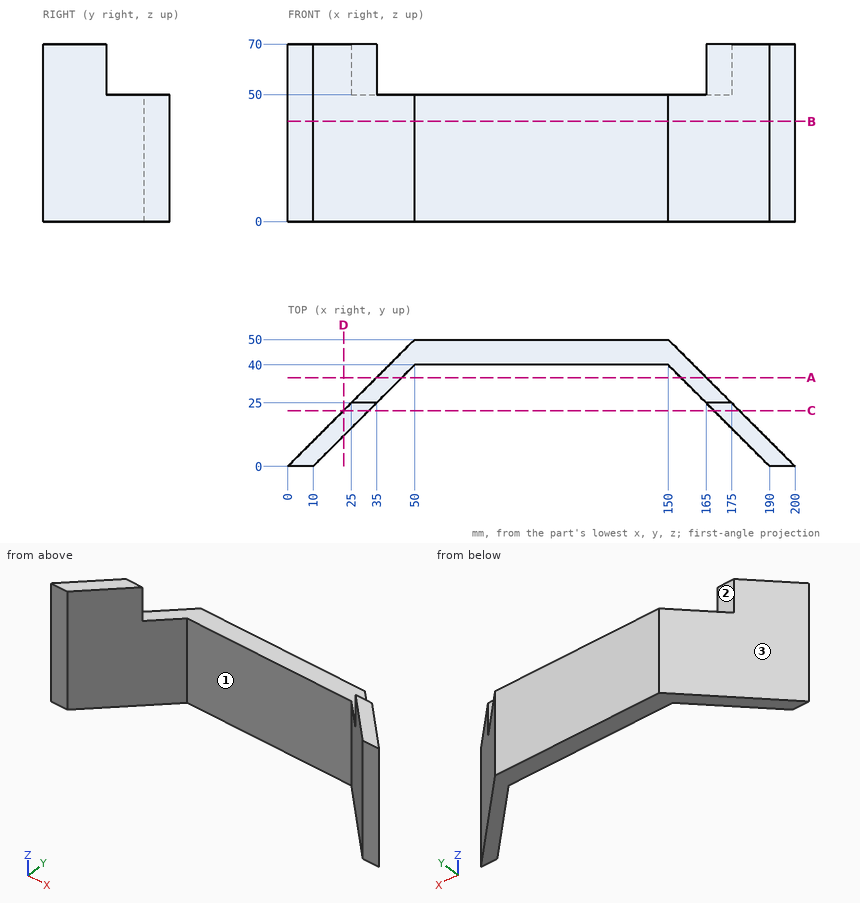
Drawing for the job (mm, zero at the part's lowest x, y, z). A direction names the side the tool comes from. Round coordinates to 2 decimals unless told otherwise and drop trailing zeros. Loops run counter-clockwise (first coordinate to the right, second up) from the corner with the lowest first, then second, coordinate; pieces in that order, holes last. Notation, with made-up numbers: (-4, -11.75) - (20, -11.75) arc R10 cw to (20, -3.75) - close; hole circle Ø2 at (0, -14). An arc over 180 degrees is marked (long way). Return JSON: item names as keys, results as strings. Group by question number.
Q1. Drill centre lines: line 1 along Y through (x, z) = (85, 26); line 2 along X through (y, z) = (21, 60); line 3 along X through (y, z) = (7.5, 9). Where is each one in solid material? Low to high. Write a range as [from, to].
Q2. Band-saw the part on D-D on x = 22. Give the cut face in (y, z).
Q3. Band-saw the part on B-B on z = 39.5. Give the cut face in (x, y), plus the area to 3 significant figures.
Q4. Flat gauge pins, fed straight in: pin 1 Ø10 at (x, z) = (115.5, 47) entering from -Y; pin 2 Ø6 at (x, z) = (165.5, 53.5) entering from +Y; pin 3 Ø1 at (x, z) = (176.5, 25) entering from -Y; pin 4 Ø12.5 at (x, y) = (102, 31.5) entering from +Z. Where does each tip first touch, or does it go through?
Q5. Band-saw the part on C-C on y = 22. Give the cut face in (x, z), plus the area to 3 significant figures.
Q6. Band-saw the part on A-A on y = 35. Give the cut face in (x, z).
Q7. Tool access for the marked faces 1, 2 and 3: list every direction of +Z, -Z, +X, -X, +Y, -Y with a clear straight run to the whole face (end or side of a thin tool).
Solutions:
{
 "1": {"line 1": "y = [40, 50]", "line 2": "x = [21, 31], [169, 179]", "line 3": "x = [7.5, 17.5], [182.5, 192.5]"},
 "2": {"outline": "(12, 0) - (22, 0) - (22, 70) - (12, 70) - close"},
 "3": {"outline": "(0, 0) - (10, 0) - (50, 40) - (150, 40) - (190, 0) - (200, 0) - (150, 50) - (50, 50) - close", "area": "1,900 mm^2"},
 "4": {"pin 1": "stops at y = 40", "pin 2": "stops at y = 25", "pin 3": "stops at y = 13", "pin 4": "passes through"},
 "5": {"outline": "(22, 0) - (32, 0) - (32, 70) - (22, 70) - close; (168, 0) - (178, 0) - (178, 70) - (168, 70) - close", "area": "1,400 mm^2"},
 "6": {"outline": "(35, 0) - (45, 0) - (45, 50) - (35, 50) - close; (155, 0) - (165, 0) - (165, 50) - (155, 50) - close"},
 "7": {"face 1": "+Z, -Z, -Y", "face 2": "+Z, +X, -X, +Y", "face 3": "+Z, -Z, -X, +Y"}
}
